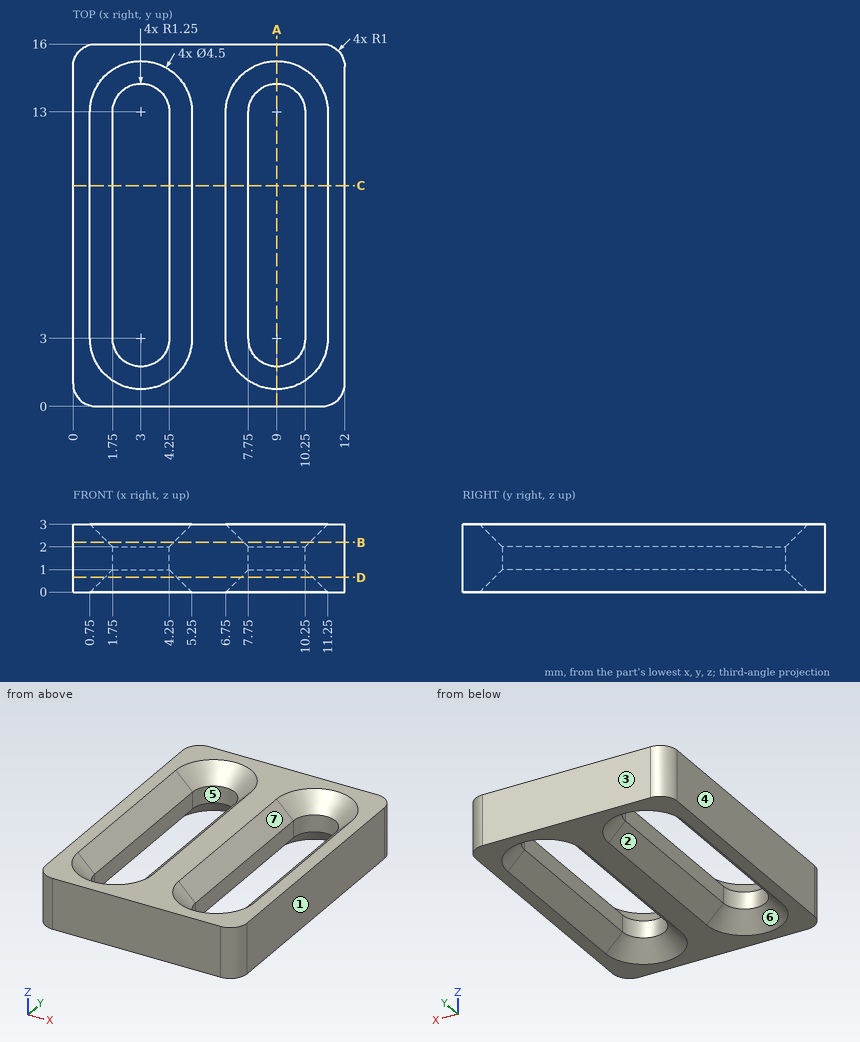
Source: three-view drawing plus pictorial views. Frame: mm from the lowest corner of the part. A direction names the side the tool comes from. Round coordinates to 2 decimals unless told otherwise and drop trailing zeros. Order: outer loops, then holes, each group sorted by start corner. A loop starts at its lowest first (then second) coordinate and runs counter-clockwise, first axis right, second up. Notation, with made-up numbers: (13, 67.5) - (69, 67.5) arc R29 ccw to (69, 106.5) - close; hole circle Ø4 at (-32.75, 6). An arc over 180 degrees is marked (long way). Use a Markdown table: item, result.
1. Section C-C on y = 9.75. Return the cut outline in (x, z), then the cut area to 3 significant figures.
Evaluation:
| item | result |
|---|---|
| outline | (0, 0) - (0.75, 0) - (1.75, 1) - (1.75, 2) - (0.75, 3) - (0, 3) - close; (4.25, 1) - (5.25, 0) - (6.75, 0) - (7.75, 1) - (7.75, 2) - (6.75, 3) - (5.25, 3) - (4.25, 2) - close; (10.25, 1) - (11.25, 0) - (12, 0) - (12, 3) - (11.25, 3) - (10.25, 2) - close |
| area | 17.0 mm^2 |
2. Section B-B on z = 2.2. Return the cut outline in (x, y), then the cut area to 3 significant figures.
Evaluation:
| item | result |
|---|---|
| outline | (0, 1) arc R1 ccw to (1, 0) - (11, 0) arc R1 ccw to (12, 1) - (12, 15) arc R1 ccw to (11, 16) - (1, 16) arc R1 ccw to (0, 15) - close; hole (1.55, 3) arc R1.45 ccw to (4.45, 3) - (4.45, 13) arc R1.45 ccw to (1.55, 13) - close; hole (7.55, 3) arc R1.45 ccw to (10.45, 3) - (10.45, 13) arc R1.45 ccw to (7.55, 13) - close |
| area | 120 mm^2 |
3. Section D-D on z = 0.65. Return the cut outline in (x, y), then the cut area to 3 significant figures.
Evaluation:
| item | result |
|---|---|
| outline | (0, 1) arc R1 ccw to (1, 0) - (11, 0) arc R1 ccw to (12, 1) - (12, 15) arc R1 ccw to (11, 16) - (1, 16) arc R1 ccw to (0, 15) - close; hole (1.4, 3) arc R1.6 ccw to (4.6, 3) - (4.6, 13) arc R1.6 ccw to (1.4, 13) - close; hole (7.4, 3) arc R1.6 ccw to (10.6, 3) - (10.6, 13) arc R1.6 ccw to (7.4, 13) - close |
| area | 111 mm^2 |
4. Mould query, pull axis X, two halves, no side actions, for the marked faces 1, 2, 3 and 4. Classes: +X half, -X half, draft (parallel to the pull), parting line (faces both ways), or undercut.
Evaluation:
| item | result |
|---|---|
| face 1 | +X half |
| face 2 | undercut |
| face 3 | draft |
| face 4 | -X half |
5. Access query for the marked faces 5, 6 and 7. Directions: +Z, -Z, +X, -X, +Y, -Y. A direction counts if a zero-diameter tool reaches every point of the face in a straight line with its end or side. Return the directions, or none.
Evaluation:
| item | result |
|---|---|
| face 5 | +Z, -Z |
| face 6 | -Z |
| face 7 | +Z |
6. Material intervals for probe 1 along X at (y, z) = (10, 1.5); probe 2 along Y at (x, z) = (3, 1.1); probe 3 along X at (y, z) = (9.25, 2.65), sorted ascending.
Evaluation:
| item | result |
|---|---|
| probe 1 | 0 to 1.75, 4.25 to 7.75, 10.25 to 12 |
| probe 2 | 0 to 1.75, 14.25 to 16 |
| probe 3 | 0 to 1.1, 4.9 to 7.1, 10.9 to 12 |
7. Section A-A on x = 9. Return the cut outline in (y, z).
Evaluation:
| item | result |
|---|---|
| outline | (0, 0) - (0.75, 0) - (1.75, 1) - (1.75, 2) - (0.75, 3) - (0, 3) - close; (14.25, 1) - (15.25, 0) - (16, 0) - (16, 3) - (15.25, 3) - (14.25, 2) - close |
